Design review of the part shown in the three views and the two pictorial views. Dimensions are in mm from the part's minimum x, y and z. A direction names the side the tool comes from. Coordinates: 2 decimals unless noted, no trailing zeros. Write each loop counter-clockwise with the first axis right and the second up, starting at its lowest first coordinate (ties: lowest second). Pieces come first, ordered by that corner, then holes.
Q1. Take a section at B-B, the plane x = 357. Write out the cut boundary in (y, z) (1 decimal).
Q2. Take a section at C-C, the plane y = 87. Write out the cut boundary in (x, z) (1 decimal), plus the area to 3 significant figures.
Q3. For L1, parallel to X at y = 94.5, z = 183.5 (1 decimal); L2, parallel to Y at x = 321, z = 217 (1 decimal), list the stretches that pass through material, from the lowest coordinate up.
Q4. For pin 1 Ø2.5 at (y, z) = (156, 256.5) entering from +X; pin 2 Ø12 at (x, z) = (224, 200) entering from -Y; pin 3 Ø1 at (y, z) = (139, 56) entering from -X, all flat-tipped, find the tip position at first contact; note any pin that passes through.
Q5. For the marked faces 1 and 2, list the 3-axis set-ups (+Z, -Z, +X, -X, +Y, -Y) from which the entire face can be reached by the end or side of a thin tool; tool diameter is ignored.
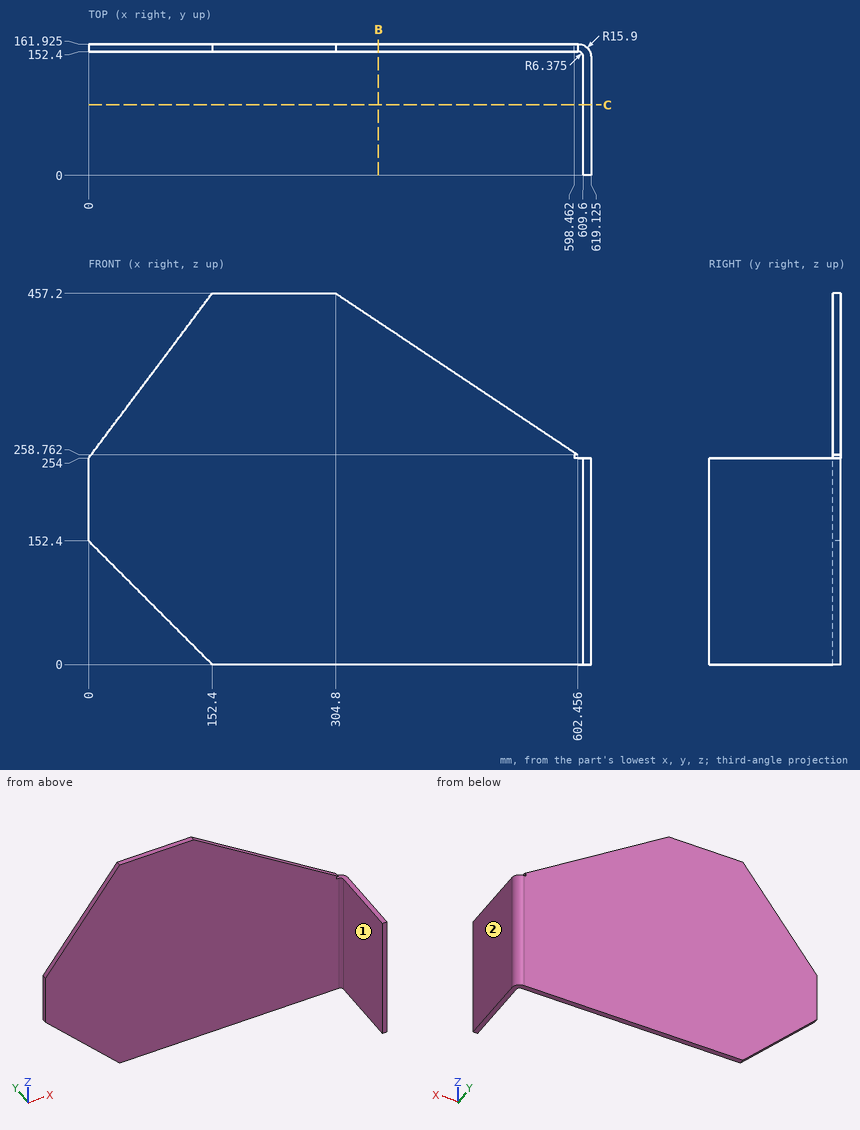
Responses:
1. outline: (152.4, 0) - (161.9, 0) - (161.9, 422.4) - (152.4, 422.4) - close
2. outline: (609.6, 0) - (619.1, 0) - (619.1, 254) - (609.6, 254) - close
2. area: 2,420 mm2
3. L1: x = 609.6 to 619.1
3. L2: y = 152.4 to 161.9
4. pin 1: stops at x = 598.46
4. pin 2: stops at y = 152.4
4. pin 3: stops at x = 609.6
5. face 1: +Z, -Z, -X, -Y
5. face 2: +Z, -Z, +X, +Y, -Y
